from build123d import *

# Parameters (mm, degrees)
PAD_DEPTH            = 37.45
SKETCH001_W          = 16.5
SKETCH001_H          = 10
PAD001_DEPTH         = 10
SKETCH002_R          = 11
PAD002_DEPTH         = 6
SKETCH003_R          = 2.545
PAD003_DEPTH         = 20
BODY_PLACEMENT_ANGLE = 90


with BuildPart() as part:
    # Sketch → Pad (new body)
    with BuildSketch(Plane.XY):
        Polygon((-21.2, 16.95), (-21.2, -16.95), (-16.95, -21.2), (16.95, -21.2), (21.2, -16.95), (21.2, 16.95), (16.95, 21.2), (-16.95, 21.2), align=None)
    extrude(amount=PAD_DEPTH)

    # Sketch001 (on Face3 of Pad) → Pad001 (join)
    with BuildSketch(Plane.XZ.offset(21.2)):
        with Locations((0, 5)):
            Rectangle(SKETCH001_W, SKETCH001_H)
    extrude(amount=PAD001_DEPTH)

    # Sketch002 (on Face5 of Pad001) → Pad002 (join)
    with BuildSketch(Plane.XY.offset(37.45)):
        Circle(SKETCH002_R)
    extrude(amount=PAD002_DEPTH)

    # Sketch003 (on Face17 of Pad002) → Pad003 (join)
    with BuildSketch(Plane.XY.offset(43.45)):
        Circle(SKETCH003_R)
    extrude(amount=PAD003_DEPTH)


with BuildPart() as part_1:
    # Body placement: moved
    add(part.part.moved(Location((-20, 0, 0))).rotate(Axis((-20, 0, 0), (0, -1, 0)), BODY_PLACEMENT_ANGLE))


solid = part_1.part
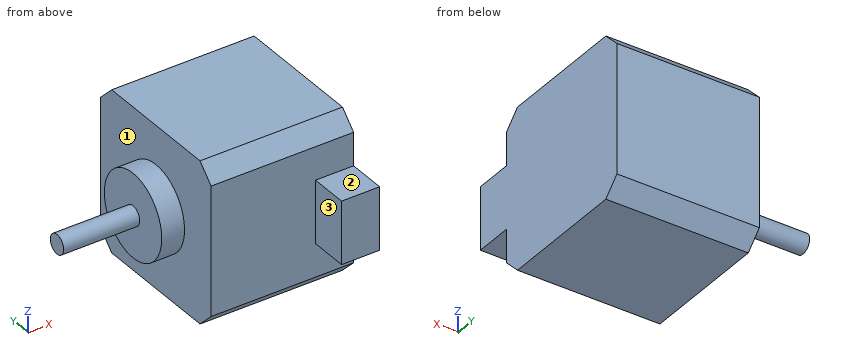
Model file for the job. Use its own axes, mm. Face numbers are marked on the shaded views. A direction names the side the tool comes from. Coordinates: 2 decimals unless noted, no trailing zeros. Write each loop counter-clockwise with the first axis right and the second up, starting at its lowest first coordinate (ties: lowest second). Pieces come first, ordered by that corner, then holes. Notation, with made-up numbers: (-16.5, 1.25) -> (9.5, 1.25) arc R10 cw to (9.5, 15.25) -> close; hole circle Ø2 at (4, 85). An arc over 180 degrees is marked (long way). One line per item, written item: value. Start each with the question number.
1) Which spindle directions (+Z, -Z, +X, -X, +Y, -Y) get a long thin tool onto all of the face, cutting with end or side? Do the marked faces 1, 2 and 3. Say none if no direction does.
2) Slice it at C-C on z = 0. Write the cut outline in (x, y) (3 decimals).
3) Flat gauge pins, fed straight in: pin 1 Ø8 at (x, z) = (-42, -7) entering from -Y; pin 2 Ø12.5 at (y, z) = (3.5, 9) entering from -X; pin 3 Ø8 at (x, y) = (-26.5, -26) entering from +Z. Where does each tip first touch, or does it go through?
4) Slice it at B-B on x = -35. Write the cut outline in (y, z).
5) Slice it at A-A on y = 0. Write the cut outline in (x, z) (3 decimals).
6) Probe probe 1 along X at (y, z) = (9.5, -11.5); probe 2 along Y at (x, z) = (-34, 1.5); probe 3 along Z at (x, y) = (-30, 17). List the from-to ranges inside material, lowest first.
7) Slice it at D-D on z = 6. Write the cut outline in (x, y), then the cut area to 3 significant figures.
Answers follow:
1. face 1: -X
1. face 2: +Z, +X, -X, -Y
1. face 3: +Z, -Z, -X, -Y
2. outline: (-83.45, -2.545) -> (-63.45, -2.545) -> (-63.45, -11) -> (-57.45, -11) -> (-57.45, -21.2) -> (-30, -21.2) -> (-30, -31.2) -> (-20, -31.2) -> (-20, 21.2) -> (-57.45, 21.2) -> (-57.45, 11) -> (-63.45, 11) -> (-63.45, 2.545) -> (-83.45, 2.545) -> close
3. pin 1: y = -21.2
3. pin 2: x = -63.45
3. pin 3: z = 8.25
4. outline: (-21.2, -16.95) -> (-16.95, -21.2) -> (16.95, -21.2) -> (21.2, -16.95) -> (21.2, 16.95) -> (16.95, 21.2) -> (-16.95, 21.2) -> (-21.2, 16.95) -> close
5. outline: (-83.45, -2.545) -> (-63.45, -2.545) -> (-63.45, -11) -> (-57.45, -11) -> (-57.45, -21.2) -> (-20, -21.2) -> (-20, 21.2) -> (-57.45, 21.2) -> (-57.45, 11) -> (-63.45, 11) -> (-63.45, 2.545) -> (-83.45, 2.545) -> close
6. probe 1: -57.45 to -20
6. probe 2: -21.2 to 21.2
6. probe 3: -21.15 to 21.15
7. outline: (-63.45, -9.22) -> (-57.45, -9.22) -> (-57.45, -21.2) -> (-30, -21.2) -> (-30, -31.2) -> (-20, -31.2) -> (-20, 21.2) -> (-57.45, 21.2) -> (-57.45, 9.22) -> (-63.45, 9.22) -> close
7. area: 1,800 mm2
